Source: CAD feature listing. Evaluate the final solid. Frame: model axes, mm. Face numbers are marked on the shaded views. A direction names the side the tool comes from. Coordinates: 2 decimals unless noted, no trailing zeros. Order: outer loops, then holes, each group sorted by start corner. A loop starts at its lowest first (then second) coordinate and runs counter-clockwise, first axis right, second up.
Item 1: Section A-A on z = 0. Return the cut outline in (x, y), then the cut area to 3 significant figures.
Item 2: Section D-D on x = 0. Return the cut outline in (y, z).
Item 3: Section C-C on x = -37. Return the cut outline in (y, z).
Item 4: Reachability of the marked faces 1 and 2 from +Z, -Z, +X, -X, +Y, -Y: full face, straight path, thin tool, end or side. Return the list, or none.
Item 5: Ray query, line 1 (Y direction, x = 49.5, z = 0); line 2 (Y direction, x = -4.25, z = 0); line 3 (Z direction, x = -43.5, y = 29). Return the intervals inside material, ascending.
Item 6: Section B-B on y = 0. Return the cut outline in (x, z), then the cut area to 3 significant figures.
Item 7: Mould query, pull axis Z, two halves, no side actions, for the marked faces 3, 4 and 5. Classes: released by +Z, released by -Z, zero draft, split by the parting line, or undercut.
Item 8: Contact query for flat-ended pins moving along their axis: P1, Ø2, axis at x = 0, y = 3.5, coming from the -Z side; P2, Ø5, axis at x = 51.5, z = -18, coming from the -Y side; P3, Ø12, axis at x = -13.5, y = 28.5, coming from the +Z side. Output: stop coordinate, or through.
from build123d import *

# Parameters (mm, degrees)
SKETCH_1_R              = 50
SKETCH_1_R_2            = 30.5
EXTRUDE_1_DEPTH         = 70
SKETCH_4_R              = 35
CUT_EXTRUDE_1_DEPTH     = 61
CUT_EXTRUDE_START       = -61
SKETCH_5_R              = 35
CUT_EXTRUDE_2_DEPTH     = 61
CHAMFER_1_SIZE          = 1.5
HOLE_WIZARD_M14_1_D     = 12
HOLE_WIZARD_M14_1_DEPTH = 38
HOLE_WIZARD_M14_1_TIP   = 3.605163714


with BuildPart() as part:
    # 草图1 → 凸台-拉伸1 (new, symmetric)
    with BuildSketch(Plane(origin=(0, 0, 0), x_dir=(0, 0, -1), z_dir=(1, 0, 0))):
        Circle(SKETCH_1_R)
        Circle(SKETCH_1_R_2, mode=Mode.SUBTRACT)
    extrude(amount=EXTRUDE_1_DEPTH, both=True)

    # 草图4 → 切除-拉伸1 (cut)
    with BuildSketch(Plane.ZY.offset(70)):
        Circle(SKETCH_4_R)
    extrude(amount=-CUT_EXTRUDE_1_DEPTH, mode=Mode.SUBTRACT)

    # 草图5 → 切除-拉伸2 (cut)
    with BuildSketch(Plane(origin=(70, 0, 0), x_dir=(0, 0, -1), z_dir=(1, 0, 0)).offset(CUT_EXTRUDE_START)):
        with Locations(Location((0, 0, 0), (0, 0, 180))):
            Circle(SKETCH_5_R)
    extrude(amount=CUT_EXTRUDE_2_DEPTH, mode=Mode.SUBTRACT)

    # 倒角1
    chamfer_1_edges = [part.edges().sort_by_distance(p)[0] for p in [
        (-70, 0, -35),
        (70, 0, -35),
        (-70, 0, 50),
        (70, 0, 50),
    ]]
    chamfer(chamfer_1_edges, length=CHAMFER_1_SIZE)

    # M14 螺纹孔1
    with Locations(Plane(origin=(0, 50, 0), x_dir=(1, 0, 0), z_dir=(0, 1, 0))):
        with Locations((0, 0)):
            Hole(HOLE_WIZARD_M14_1_D / 2, depth=HOLE_WIZARD_M14_1_DEPTH)
            with Locations((0, 0, -(HOLE_WIZARD_M14_1_DEPTH + HOLE_WIZARD_M14_1_TIP / 2))):  # 118° drill point
                Cone(0, HOLE_WIZARD_M14_1_D / 2, HOLE_WIZARD_M14_1_TIP, mode=Mode.SUBTRACT)


solid = part.part
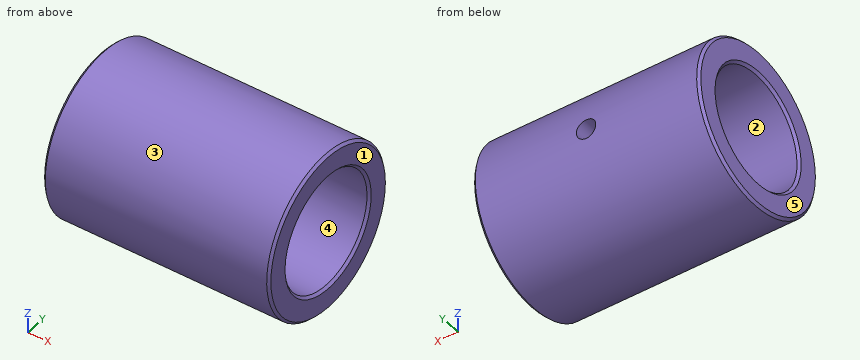
Answer list:
1. outline: (-70, -48.5) - (-68.5, -50) - (68.5, -50) - (70, -48.5) - (70, -36.5) - (68.5, -35) - (9, -35) - (9, -30.5) - (-9, -30.5) - (-9, -35) - (-68.5, -35) - (-70, -36.5) - close; (-70, 36.5) - (-68.5, 35) - (-9, 35) - (-9, 30.5) - (-6, 30.5) - (-6, 50) - (-68.5, 50) - (-70, 48.5) - close; (6, 30.5) - (9, 30.5) - (9, 35) - (68.5, 35) - (70, 36.5) - (70, 48.5) - (68.5, 50) - (6, 50) - close
1. area: 4,120 mm2
2. outline: (29.9, -6) arc R30.5 cw (long way) to (29.9, 6) - (49.64, 6) arc R50 ccw (long way) to (49.64, -6) - close
3. outline: circle Ø100 at (0, 0); hole circle Ø70 at (0, 0)
4. face 1: +Z, -Z, +X, +Y, -Y
4. face 2: -X
5. line 1: y = -50 to -35, 35 to 50
5. line 2: y = -50 to -30.5
5. line 3: z = -40.73 to -19.6, 19.6 to 40.73
6. outline: (-70, -48.5) - (-68.5, -50) - (68.5, -50) - (70, -48.5) - (70, -36.5) - (68.5, -35) - (9, -35) - (9, -30.5) - (-9, -30.5) - (-9, -35) - (-68.5, -35) - (-70, -36.5) - close; (-70, 36.5) - (-68.5, 35) - (-9, 35) - (-9, 30.5) - (9, 30.5) - (9, 35) - (68.5, 35) - (70, 36.5) - (70, 48.5) - (68.5, 50) - (-68.5, 50) - (-70, 48.5) - close
6. area: 4,350 mm2
7. face 3: split by the parting line
7. face 4: undercut
7. face 5: zero draft
8. P1: stops at z = -49.94
8. P2: stops at y = -47.54
8. P3: stops at z = 44.65
